from build123d import *

# Parameters (mm, degrees)
F0_W     = 22
F0_H     = 22
F0_R     = 1.35
F0_R_2   = 1.9
F1_DEPTH = 8
F2_W     = 8.2
F2_H     = 16.4
F2_R     = 1.9
F3_DEPTH = 6
F4_DEPTH = 4
F5_R     = 1.24999


# Not quite as in the source:
# - a fillet or chamfer is up to 0.001 mm smaller than in the source, because OpenCascade refuses the exact size


with BuildPart() as f1:
    # F0 (on Top) → F1 (new body)
    with BuildSketch(Plane.XY):
        Rectangle(F0_W, F0_H)
        with Locations((-8, -8)):
            Circle(F0_R, mode=Mode.SUBTRACT)
        with Locations((8, -8)):
            Circle(F0_R, mode=Mode.SUBTRACT)
        with Locations((0, -3)):
            Circle(F0_R_2, mode=Mode.SUBTRACT)
        with Locations((-8, 8)):
            Circle(F0_R, mode=Mode.SUBTRACT)
        with Locations((0, 3)):
            Circle(F0_R_2, mode=Mode.SUBTRACT)
        with Locations((8, 8)):
            Circle(F0_R, mode=Mode.SUBTRACT)
    extrude(amount=F1_DEPTH)

    # F2 (on face) → F3 (cut)
    with BuildSketch(Plane.XY.offset(8)):
        Rectangle(F2_W, F2_H)
        with Locations((0, -3)):
            Circle(F2_R, mode=Mode.SUBTRACT)
        with Locations((0, 3)):
            Circle(F2_R, mode=Mode.SUBTRACT)
    extrude(amount=-F3_DEPTH, mode=Mode.SUBTRACT)

    # F2 (on face) → F4 (cut)
    with BuildSketch(Plane.XY.offset(8)):
        with BuildLine():
            ThreePointArc((-5.5, 8), (-6.232233047, 6.232233047), (-8, 5.5))
            Line((-8, 5.5), (-9.25, 5.5))
            Line((-9.25, 5.5), (-9.25, -5.5))
            Line((-9.25, -5.5), (-8, -5.5))
            ThreePointArc((-8, -5.5), (-6.232233047, -6.232233047), (-5.5, -8))
            Line((-5.5, -8), (-5.5, -9.25))
            Line((-5.5, -9.25), (5.5, -9.25))
            Line((5.5, -9.25), (5.5, -8))
            ThreePointArc((5.5, -8), (6.232233047, -6.232233047), (8, -5.5))
            Line((8, -5.5), (9.25, -5.5))
            Line((9.25, -5.5), (9.25, 5.5))
            Line((9.25, 5.5), (8, 5.5))
            ThreePointArc((8, 5.5), (6.232233047, 6.232233047), (5.5, 8))
            Line((5.5, 8), (5.5, 9.25))
            Line((5.5, 9.25), (-5.5, 9.25))
            Line((-5.5, 9.25), (-5.5, 8))
        make_face()
        Rectangle(F2_W, F2_H, mode=Mode.SUBTRACT)
    extrude(amount=-F4_DEPTH, mode=Mode.SUBTRACT)

    # F5 (radius 1.25 in the source; OpenCascade refuses exactly that, so slightly less here)
    f5_edges = [f1.edges().sort_by_distance(p)[0] for p in [
        (-9.25, 5.5, 6),
        (-5.5, 9.25, 6),
        (5.5, 9.25, 6),
        (9.25, 5.5, 6),
        (-9.25, -5.5, 6),
        (-5.5, -9.25, 6),
        (5.5, -9.25, 6),
        (9.25, -5.5, 6),
    ]]
    fillet(f5_edges, radius=F5_R)


solid = f1.part
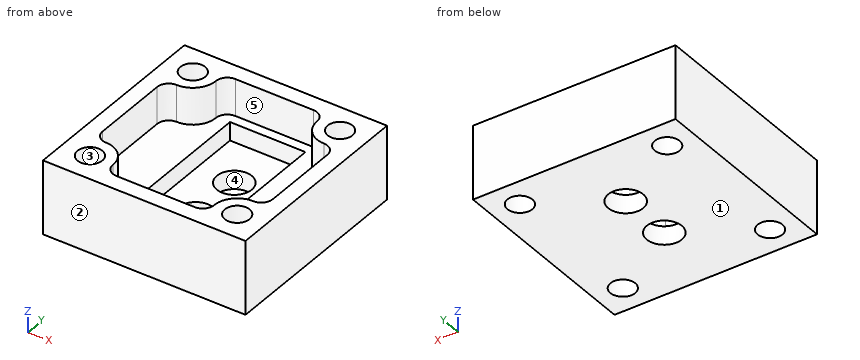
Could you check a few things on this model? Use its own coordinates, in mm. Face numbers are marked on the shaded views. A direction names the side the tool comes from. Round coordinates to 2 decimals unless told otherwise and drop trailing zeros. Order: outer loops, then holes, each group sorted by start corner. A loop starts at its lowest first (then second) coordinate and runs counter-clockwise, first axis right, second up.
Q1. Which directions (+Z, -Z, +X, -X, +Y, -Y) give clear straight access to the entire face, cutting with the end or side of a thin tool? Please do the marked faces 4 and 5.
Geometry says:
face 4: +Z, -Z
face 5: +Z
Q2. Imagine slicing it at B-B, the plane y = 3. List the corners of the cut face in (x, z) for me, then the cut area to 3 significant figures.
Geometry says:
outline: (-11, 0) - (-1.9, 0) - (-1.9, 2) - (-4.1, 2) - (-4.1, 4) - (-9.25, 4) - (-9.25, 8) - (-11, 8) - close; (1.9, 0) - (11, 0) - (11, 8) - (9.25, 8) - (9.25, 4) - (4.1, 4) - (4.1, 2) - (1.9, 2) - close
area: 78.0 mm2
Q3. Imagine slicing it at D-D, the plane y = -0.75. List the corners of the cut face in (x, z) for me.
Geometry says:
outline: (-11, 0) - (11, 0) - (11, 8) - (9.25, 8) - (9.25, 4) - (4.1, 4) - (4.1, 2) - (-4.1, 2) - (-4.1, 4) - (-9.25, 4) - (-9.25, 8) - (-11, 8) - close
Q4. Thinking about a two-plate mould opening in Y: for the marked faces 1, 2 and 3, which applies, released by +Y, released by -Y, zero draft, split by the parting line, or undercut?
Geometry says:
face 1: zero draft
face 2: released by -Y
face 3: undercut
Q5. I'm going to push flat-ended pins straight in: P1, Ø2, axis at x = -8, y = 8, coming from the -Z side; P2, Ø1, axis at x = 4.5, y = -8, coming from the +Z side. Where does each tip first touch, or does it pass through?
Geometry says:
P1: passes through
P2: stops at z = 4
Q6. Imagine slicing it at A-A, the plane x = 0. List the corners of the cut face in (y, z) for me.
Geometry says:
outline: (-11, 0) - (-4.9, 0) - (-4.9, 2) - (-8.2, 2) - (-8.2, 4) - (-9.25, 4) - (-9.25, 8) - (-11, 8) - close; (-1.1, 0) - (1.1, 0) - (1.1, 2) - (-1.1, 2) - close; (4.9, 0) - (11, 0) - (11, 8) - (9.25, 8) - (9.25, 4) - (8.2, 4) - (8.2, 2) - (4.9, 2) - close
Q7. Imagine slicing it at C-C, the plane z = 4.5. State how many separate pieces and enclosed holes the cut face has, then the cut area to 3 significant figures.
Geometry says:
separate pieces: 1
enclosed holes: 5
area: 172 mm2
Q8. Please list where these lines run through material, in increasing order: probe 1 along Y at (x, z) = (0, 1.4); probe 2 along Y at (x, z) = (8, 1.75); probe 3 along X at (y, z) = (5, 3.75).
Geometry says:
probe 1: y = -11 to -4.9, -1.1 to 1.1, 4.9 to 11
probe 2: y = -11 to -9.35, -6.65 to 6.65, 9.35 to 11
probe 3: x = -11 to -4.1, 4.1 to 11
